Could you check a few things on this model? Use its own coordinates, in mm. A direction names the side the tool comes from. Give positions to 0.01 mm unless a question says otherwise; leave off trailing zeros. Loops run counter-clockwise (first coordinate to the right, second up) from the corner with the lowest first, then second, coordinate; pieces in that order, holes last. Notation, with made-up numbers: M 3,19.5 L 36,19.5 A34 ccw 36,50.5 Z; hole C -20,78.25 d11. An arc over 180 degrees is marked long. Use a Markdown table: item, result. Add a question column.
1) Suppose I cut it at A-A on x = 0. List the corners of the cut face in (y, z) for me.
2) Suppose I cut it at C-C on y = 0.85. List the corners of the cut face in (x, z) for me.
3) Will these pins go through, and if not, where does the flat tip stop? pin 1 Ø0.7 at (x, z) = (-3.5, -3) entering from +Y; pin 2 Ø0.9 at (x, y) = (-3.5, 2.5) entering from -Z; pin 3 Ø3 at (x, z) = (-1, -9) entering from +Y.
4) Suppose I cut it at D-D on z = -11. List the corners of the cut face in (x, y) for me.
5) Which directions (+Z, -Z, +X, -X, +Y, -Y) give clear straight access to the entire face, cutting with the end or side of a thin tool? Please do faces 4 (the flat face through (3.3, 2.2, -5.9)), 5 (the flat face through (3.2, 2.3, -9.6)), 6 (the flat face through (-3.3, 2.2, -11.8)), 7 (the flat face through (-3.3, 1.95, -2.7)), 8 (the flat face through (-3.3, 2.2, -5.9)).
6) Suppose I cut it at B-B on z = -2.75. List the corners of the cut face in (x, y) for me, and give its area (3 significant figures).
7) We'd pull the mould along X, two halves only. Please class faces 1 (the flat face through (2.63, 1.6, 0)), 2 (the cylindrical face through (-0.39, 0.343, -4.846)), 3 (the flat face through (3.29, 2.56, -8.86)): +X half, -X half, draft (parallel to the pull), parting line (faces both ways), or undercut.
8) If I drill on line 1 along Y through (x, z) = (0, -3); line 2 along Y through (x, z) = (2.5, -6.75); line 3 along Y through (x, z) = (1, -4.75), over which ranges is the centre line in solid material (lowest first)? Write a range as [from, to].
```python
from build123d import *

# Parameters (mm, degrees)
SKETCH_1_W          = 5.8
SKETCH_1_H          = 12.4
EXTRUDE_1_DEPTH     = 4.2
SKETCH_2_R          = 2.5
EXTRUDE_2_DEPTH     = 2.5
SKETCH_4_W          = 1
SKETCH_4_H          = 0.25
EXTRUDE_4_DEPTH     = 0.9
SKETCH_5_R          = 1.8
CUT_EXTRUDE_1_DEPTH = 17.050233643
SKETCH_6_W          = 1.5
SKETCH_6_H          = 1
EXTRUDE_5_DEPTH     = 0.8
CUT_EXTRUDE_2_DEPTH = 1.5


with BuildPart() as part:
    # 草图1 → 凸台-拉伸1 (new body)
    with BuildSketch(Plane(origin=(0, 0, 0), x_dir=(1, 0, 0), z_dir=(0, 1, 0))):
        with Locations((0, 6.2)):
            Rectangle(SKETCH_1_W, SKETCH_1_H)
    extrude(amount=EXTRUDE_1_DEPTH)

    # 草图2 → 凸台-拉伸2 (add)
    with BuildSketch(Plane.XY):
        with Locations(Location((0, 2.1, 0), (0, 0, 122.859880379))):
            Circle(SKETCH_2_R)
    extrude(amount=EXTRUDE_2_DEPTH)

    # 草图4 → 凸台-拉伸4 (add)
    with BuildSketch(Plane(origin=(2.9, 0, 0), x_dir=(0, 0, -1), z_dir=(1, 0, 0))):
        with Locations((2.7, 2.075)):
            Rectangle(SKETCH_4_W, SKETCH_4_H)
        with Locations((5.9, 2.075)):
            Rectangle(SKETCH_4_W, SKETCH_4_H)
        with Locations((11.8, 2.075)):
            Rectangle(SKETCH_4_W, SKETCH_4_H)
    extrude_4 = extrude(amount=EXTRUDE_4_DEPTH)

    # 草图5 → 切除-拉伸1 (cut, through all)
    with BuildSketch(Plane.XY.offset(2.5)):
        with Locations((0, 2.1)):
            Circle(SKETCH_5_R)
    extrude(amount=-CUT_EXTRUDE_1_DEPTH, mode=Mode.SUBTRACT)

    # 草图6 → 凸台-拉伸5 (add)
    with BuildSketch(Plane(origin=(2.9, 0, 0), x_dir=(0, 0, -1), z_dir=(1, 0, 0))):
        with Locations((8.85, 2.45)):
            Rectangle(SKETCH_6_W, SKETCH_6_H)
    extrude_5 = extrude(amount=EXTRUDE_5_DEPTH)

    # 草图7 → 切除-拉伸2 (cut)
    with BuildSketch(Plane(origin=(0, 0, -9.6), x_dir=(-1, 0, 0), z_dir=(0, 0, -1))):
        Polygon((-3.7, 2.95), (-2.9, 2.95), (-3.7, 2.15), align=None)
    cut_extrude_2 = extrude(amount=-CUT_EXTRUDE_2_DEPTH, mode=Mode.SUBTRACT)

    # 镜向1: 凸台-拉伸4, 凸台-拉伸5, 切除-拉伸2 across plane
    add(extrude_4.mirror(Plane(origin=(0, 0, 0), x_dir=(0, 0, 1), z_dir=(1, 0, 0))))
    add(extrude_5.mirror(Plane(origin=(0, 0, 0), x_dir=(0, 0, 1), z_dir=(1, 0, 0))))
    add(cut_extrude_2.mirror(Plane(origin=(0, 0, 0), x_dir=(0, 0, 1), z_dir=(1, 0, 0))), mode=Mode.SUBTRACT)


solid = part.part
```
Answer block:
| question | item | result |
|---|---|---|
| 1 | outline | M -0.4,0 L 0,0 L 0,-12.4 L 0.3,-12.4 L 0.3,2.5 L -0.4,2.5 Z; M 3.9,-12.4 L 4.2,-12.4 L 4.2,0 L 4.6,0 L 4.6,2.5 L 3.9,2.5 Z |
| 2 | outline | M -2.9,-12.4 L -1.3,-12.4 L -1.3,2.5 L -2.17,2.5 L -2.17,0 L -2.9,0 Z; M 1.3,-12.4 L 2.9,-12.4 L 2.9,0 L 2.17,0 L 2.17,2.5 L 1.3,2.5 Z |
| 3 | pin 1 | stops at y = 2.2 |
| 3 | pin 2 | stops at z = -12.3 |
| 3 | pin 3 | stops at y = 4.2 |
| 4 | outline | M -2.9,0 L 2.9,0 L 2.9,4.2 L -2.9,4.2 Z; hole C 0,2.1 d3.6 |
| 5 | face 4 | +Z, +X, +Y |
| 5 | face 5 | +X, +Y, -Y |
| 5 | face 6 | -Z, -X, +Y |
| 5 | face 7 | +Z, -Z, -X, -Y |
| 5 | face 8 | +Z, -X, +Y |
| 6 | outline | M -3.8,1.95 L -2.9,1.95 L -2.9,0 L 2.9,0 L 2.9,1.95 L 3.8,1.95 L 3.8,2.2 L 2.9,2.2 L 2.9,4.2 L -2.9,4.2 L -2.9,2.2 L -3.8,2.2 Z; hole C 0,2.1 d3.6 |
| 6 | area | 14.6 mm^2 |
| 7 | face 1 | draft |
| 7 | face 2 | undercut |
| 7 | face 3 | +X half |
| 8 | line 1 | y = [0, 0.3], [3.9, 4.2] |
| 8 | line 2 | y = [0, 4.2] |
| 8 | line 3 | y = [0, 0.6], [3.6, 4.2] |
